Autodesk Inventor part; units mm, degrees
ref_plane "YZ Plane" through (0, 0, 0) normal (1, 0, 0) x (0, 1, 0)
ref_plane "XZ Plane" through (0, 0, 0) normal (0, 1, 0) x (-1, 0, 0)
ref_plane "XY Plane" through (0, 0, 0) normal (0, 0, 1) x (1, 0, 0)
sketch "Sketch1" plane through (0, 0, 0) normal (1, 0, 0) x (0, 1, 0)
  line L0 (30, 0) -> (35, 0)
  line L1 (35, 0) -> (35, 3)
  line L2 (35, 3) -> (40, 3)
  line L3 (40, 3) -> (40, 18)
  line L4 (35, 23) -> (-5, 23)
  line L5 (-10, 18) -> (-10, 3)
  line L6 (-10, 3) -> (-5, 3)
  line L7 (-5, 3) -> (-5, 0)
  line L8 (-5, 0) -> (0, 0)
  line L9 (0, 0) -> (0, 15)
  line L10 (0, 15) -> (30, 15)
  line L11 (30, 15) -> (30, 0)
  arc A0 (-5, 23) -> (-10, 18) centre (-5, 18) ccw
  arc A1 (40, 18) -> (35, 23) centre (35, 18) ccw
  point P0 (-10, 23)
  dimension "d0" = 5
  dimension "d1" = 3
  dimension "d2" = 5
  dimension "d3" = 20
  dimension "d4" = 30
  dimension "d5" = 12
  dimension "d6" = 5
  dimension "d7" = 3
  dimension "d8" = 5
  dimension "d9" = 5
extrude "Extrusion1" add sketch "Sketch1" along normal blind 3
sketch "Sketch3" plane through (3, 0, 0) normal (1, 0, 0) x (0, 0, -1)
  line L0 (0, 0) -> (-15, 0)
  line L1 (-15, 0) -> (-15, 30)
  line L2 (-15, 30) -> (0, 30)
  circle A0 centre (-9, 32.5) radius 1.5
  circle A1 centre (-9, -2.5) radius 1.5
  dimension "d12" = 3
  dimension "d14" = 3
  dimension "d15" = 6
  dimension "d16" = 6
  dimension "d17" = 2.5
  dimension "d18" = 2.5
extrude "Extrusion2" cut sketch "Sketch3" against normal blind 3
properties part number "Servo Mount 080113"
Build history of the part. All positions in model axes, mm. A direction names the side the tool comes from. Coordinates: 2 decimals unless noted, no trailing zeros. Write each loop counter-clockwise with the first axis right and the second up, starting at its lowest first coordinate (ties: lowest second). Pieces come first, ordered by that corner, then holes.
(1) Cut at A-A on x = 0.6. List the corners of the cut face in (y, z), and give its area (3 significant figures).
(2) Cut at C-C on y = 32.5. List the corners of the cut face in (x, z), and give its area (3 significant figures).
(3) Mould opens along Y. For faces 1 (the flat face through (3, 15, 17)), 2 (the flat face through (1, -5, 2)), 3 (the flat face through (1, 15, 15)) say: pulls with the +Y half, pulls with the -Y half, needs draft (parallel to the pull), parting line crosses it, or undercut.
(4) Drill centre lines: line 1 (Y direction, x = 1.9, z = 14.25); line 2 (Z direction, x = 2.5, y = -2); line 3 (Z direction, x = 1.25, y = 23.5). Where is each one in solid material? Low to high.
(5) Pin check, flat tips, straight feed: pin 1 Ø2.5 at (y, z) = (32.5, 9) entering from -X; pin 2 Ø0.9 at (x, z) = (1, 2) entering from -Y. Stop position of each tip, or through.
(6) 3-axis set-ups, long thin cutter, end or side, ignore diameter. For faces 4 (the flat face through (1, 0, 7)), 5 (the flat face through (0, 15, 17)), 6 (the flat face through (1, 37, 3)), 7 (the flat face through (1, -8, 3)), 8 (the flat face through (1, 15, 23)): which of +Z, -Z, +X, -X, +Y, -Y reach the whole face in a straight line?
(7) Cut at D-D on z = 14. List the corners of the cut face in (x, y), and give its area (3 significant figures).
(8) Cut at B-B on z = 9. List the corners of the cut face in (x, y).
Working result:
1. outline: (-10, 3) - (-5, 3) - (-5, 0) - (0, 0) - (0, 15) - (30, 15) - (30, 0) - (35, 0) - (35, 3) - (40, 3) - (40, 18) arc R5 ccw to (35, 23) - (-5, 23) arc R5 ccw to (-10, 18) - close; hole circle Ø3 at (-2.5, 9); hole circle Ø3 at (32.5, 9)
1. area: 645 mm2
2. outline: (0, 0) - (3, 0) - (3, 7.5) - (0, 7.5) - close; (0, 10.5) - (3, 10.5) - (3, 23) - (0, 23) - close
2. area: 60.0 mm2
3. face 1: needs draft
3. face 2: pulls with the -Y half
3. face 3: undercut
4. line 1: y = -10 to 0, 30 to 40
4. line 2: z = 0 to 7.59, 10.41 to 23
4. line 3: z = 15 to 23
5. pin 1: passes through
5. pin 2: stops at y = -5
6. face 4: -Z, +X, -X
6. face 5: +Z, -Z, -X, +Y, -Y
6. face 6: -Z, +X, -X, +Y
6. face 7: -Z, +X, -X, -Y
6. face 8: +Z, +X, -X, +Y, -Y
7. outline: (0, -10) - (3, -10) - (3, 0) - (0, 0) - close; (0, 30) - (3, 30) - (3, 40) - (0, 40) - close
7. area: 60.0 mm2
8. outline: (0, -10) - (3, -10) - (3, -4) - (0, -4) - close; (0, -1) - (3, -1) - (3, 0) - (0, 0) - close; (0, 30) - (3, 30) - (3, 31) - (0, 31) - close; (0, 34) - (3, 34) - (3, 40) - (0, 40) - close
